Geometry: final body of the model. Coordinates: model frame, mm. Face numbers are marked on the shaded views. A direction names the side the tool comes from. Round coordinates to 2 decimals unless told otherwise and drop trailing zeros. Write each loop counter-clockwise with the first axis right and the second up, starting at its lowest first coordinate (ties: lowest second). Pieces come first, ordered by that corner, then holes. Notation, with made-up numbers: (-30.5, -1.75) - (12.5, -1.75) arc R18 ccw to (12.5, 24.25) - close; hole circle Ø2 at (85, 8.25). An arc over 180 degrees is marked (long way). Write each question's results on one line, items separated by ' | '.
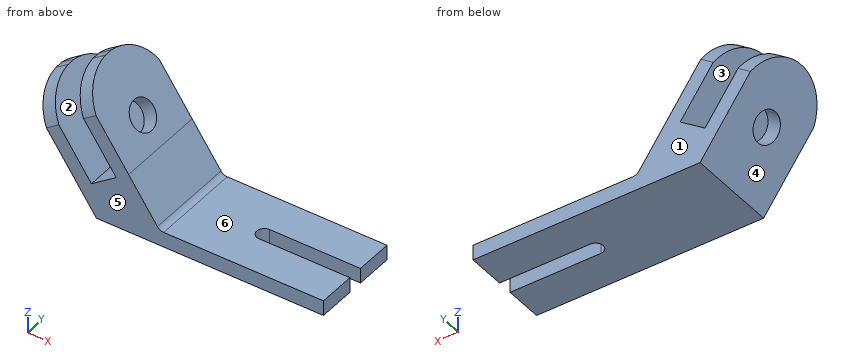
from build123d import *

# Parameters (mm, degrees)
F1_DEPTH = 60
F3_DEPTH = 77.588705
F4_R     = 10
F5_DEPTH = 52.1
F7_DEPTH = 25
F8_R     = 5


with BuildPart() as f1:
    # F0 (on Front) → F1 (new body)
    with BuildSketch(Plane.XZ):
        Polygon((-120.213985, -34.176537), (29.786015, -34.176537), (29.786015, -24.176537), (-78.385077, -24.176537), (-98.919432, 5.149562), (-133.334018, 54.298684), (-141.525538, 48.56292), (-107.110952, -0.586203), (-123.493993, -12.057731), (-157.908579, 37.091391), (-166.1001, 31.355627), align=None)
    extrude(amount=F1_DEPTH)

    # F2 (on face) → F3 (cut, through all)
    with BuildSketch(Plane(origin=(-63.956432, 0, -44.782776), x_dir=(0, 1, 0), z_dir=(0.819152, 0, 0.573576))):
        with BuildLine():
            ThreePointArc((-60, 80.946133), (-29.664459, 121.080285), (0, 80.447599))
            Line((0, 80.447599), (29.212171, 131.16917))
            Line((29.212171, 131.16917), (-70.869207, 149.550825))
            Line((-70.869207, 149.550825), (-73.535636, 96.864909))
            Line((-73.535636, 96.864909), (-60, 80.946133))
        make_face()
    extrude(amount=-F3_DEPTH, mode=Mode.SUBTRACT)

    # F4 (on face) → F5 (cut)
    with BuildSketch(Plane(origin=(-63.956432, 0, -44.782776), x_dir=(0, 1, 0), z_dir=(0.819152, 0, 0.573576))):
        with Locations((-30, 81.155573)):
            Circle(F4_R)
    extrude(amount=-F5_DEPTH, mode=Mode.SUBTRACT)

    # F6 (on face) → F7 (cut)
    with BuildSketch(Plane.XY.offset(-24.176537)):
        with BuildLine():
            ThreePointArc((-30.213985, -35), (-26.678451, -33.535534), (-25.213985, -30))
            ThreePointArc((-25.213985, -30), (-26.678451, -26.464466), (-30.213985, -25))
            ThreePointArc((-30.213985, -25), (-35.213985, -30), (-30.213985, -35))
        make_face()
        with BuildLine():
            ThreePointArc((-30.213985, -25), (-26.678451, -26.464466), (-25.213985, -30))
            ThreePointArc((-25.213985, -30), (-26.678451, -33.535534), (-30.213985, -35))
            Line((-30.213985, -35), (33.633854, -35))
            Line((33.633854, -35), (34.827039, -25))
            Line((34.827039, -25), (-30.213985, -25))
        make_face()
    extrude(amount=-F7_DEPTH, mode=Mode.SUBTRACT)

    # F8
    f8_edges = [f1.edges().sort_by_distance(p)[0] for p in [
        (-78.385077, -30, -24.176537),
    ]]
    fillet(f8_edges, radius=F8_R)


solid = f1.part
Q1. Mould query, pull axis Z, two halves, no side actions, for the marked faces 3, 4, 5 and 6. Classes: pulls with the +Z half, pulls with the -Z half, needs draft (parallel to the pull), parting line crosses it, or undercut.
Answer block:
face 3: undercut | face 4: pulls with the -Z half | face 5: needs draft | face 6: pulls with the +Z half
Q2. Section query C-C, the plane z = -26. Return loops of the section in (x, y).
Answer block:
outline: (-125.94, -60) - (29.79, -60) - (29.79, -35) - (-30.21, -35) arc R5 cw to (-30.21, -25) - (29.79, -25) - (29.79, 0) - (-125.94, 0) - close
Q3. Section query B-B, the plane y = -30. Return loops of the section in (x, z).
Answer block:
outline: (-166.1, 31.36) - (-149.01, 6.94) - (-140.82, 12.68) - (-157.91, 37.09) - close; (-141.53, 48.56) - (-124.43, 24.15) - (-116.24, 29.89) - (-133.33, 54.3) - close; (-137.54, -9.44) - (-120.21, -34.18) - (-35.21, -34.18) - (-35.21, -24.18) - (-75.78, -24.18) arc R5 cw to (-79.88, -22.04) - (-104.77, 13.5) - (-112.96, 7.77) - (-107.11, -0.59) - (-123.49, -12.06) - (-129.34, -3.7) - close
Q4. Access query for the marked faces 1 and 2. Directions: +Z, -Z, +X, -X, +Y, -Y. A direction counts if a zero-diameter tool reaches every point of the face in a straight line with its end or side. Return the directions, or none.
Answer block:
face 1: +Z, -Z, +X, -X, +Y | face 2: +Y, -Y
Q5. Pin query (flat end, axial travel): pin 1 (18 mm diameter, centred on x = -17.5, y = -29, fed in from +Z); pin 2 (1.5 mm diameter, centred on x = -133, y = -36.5, fed in from +Z); pin 3 (10 mm diameter, centred on y = -29, z = -18, fed in from +X). Return the tip coordinate at first contact, or that it passes through.
Answer block:
pin 1: z = -24.18 | pin 2: z = 53.95 | pin 3: x = -79
Q6. Section query A-A, the plane x = 2. Return loops of the section in (y, z), plus the area to 3 significant figures.
Answer block:
outline: (-60, -34.18) - (-35, -34.18) - (-35, -24.18) - (-60, -24.18) - close; (-25, -34.18) - (0, -34.18) - (0, -24.18) - (-25, -24.18) - close | area: 500 mm2
Q7. Ray query, line 1 along Z through (x, y) = (-45, -34.5); line 2 along Z through (x, y) = (-124.5, -32.5); line 3 along X through (y, z) = (-54.5, 2). Return the intervals inside material, ascending.
Answer block:
line 1: -34.18 to -24.18 | line 2: -28.06 to -10.62, 24.25 to 41.68 | line 3: -145.55 to -133.34, -108.92 to -96.71
Q8. Section query D-D, the plane x = -64.5. Return loops of the section in (y, z), plus the area to 3 significant figures.
Answer block:
outline: (-60, -34.18) - (0, -34.18) - (0, -24.18) - (-60, -24.18) - close | area: 600 mm2
